Autodesk Inventor part; units mm, degrees
ref_plane "YZ Plane" through (0, 0, 0) normal (1, 0, 0) x (0, 1, 0)
ref_plane "XZ Plane" through (0, 0, 0) normal (0, 1, 0) x (-1, 0, 0)
ref_plane "XY Plane" through (0, 0, 0) normal (0, 0, 1) x (1, 0, 0)
sketch "草圖1" plane through (0, 0, 0) normal (0, 0, 1) x (1, 0, 0)
  circle A0 centre (0, 0) radius 32
  dimension "d0" = 64
extrude "擠出1" add sketch "草圖1" along normal blind 4.5
sketch "草圖2" plane through (0, 0, 4.5) normal (0, 0, 1) x (1, 0, 0)
  point P0 (0, 0)
  point P1 (0, 0)
hole "孔1" at (0, 0, 4.5) direction (0, 0, -1) diameter 30 end through all
sketch "草圖3" plane through (0, 0, 4.5) normal (0, 0, 1) x (1, 0, 0)
  circle A0 centre (15, 0) radius 2.15
  point P0 (0, 0)
  dimension "d10" = 0
  dimension "d11" = 4.3
  dimension "d12" = 15
extrude "擠出2" cut sketch "草圖3" against normal blind 20
pattern_circular "環形陣列1" count 2 over 360 about axis through (0, 0, -86.1215) along (0, 0, 1) of "擠出2"
properties part number "銅墊塊-50T"
Read the model definition and answer for the solid it produces. Units are mm, in the model's axes. A direction names the side the tool comes from. Round coordinates to 2 decimals unless told otherwise and drop trailing zeros. Write each loop counter-clockwise with the first axis right and the second up, starting at its lowest first coordinate (ties: lowest second). Pieces come first, ordered by that corner, then holes. Notation, with made-up numbers: (43, -14.5) - (66, -14.5) arc R29 ccw to (66, 5.5) - close; hole circle Ø1 at (-32.75, -29.75). An arc over 180 degrees is marked (long way). One line per question, with ' | ' between items. Start each with the question number.
1. For a pull along X with two mould halves and no side action, classify faces 3 (the face through (-17.15, 0.05, 2.28)), 4 (the face through (14, -7, 0)), 5 (the face through (-6.94, 31.24, 2.22)), 6 (the face through (0, -15, 2)) as +X half, -X half, draft (parallel to the pull), parting line (faces both ways), or undercut.
2. Section C-C (z = 1.85) is taken. Determine the outline of the cut face in (x, y), and give its area (3 significant figures).
3. This flat-tipped pin is pushed along its axis until it touches: pin 1 (1.5 mm diameter, centred on x = 11.5, z = 3.5, fed in from +Y). Where does it stop, or does it pass through?
4. For faces 1 (the face through (0, 15, 2)), 2 (the face through (14, -7, 4.5)), determine the directions among +Z, -Z, +X, -X, +Y, -Y from which every point of the face is accessible in a straight line to the end or side of a thin tool.
5. Section A-A (y = 0) is taken. Determine the outline of the cut face in (x, z), and give its area (3 significant figures).
6. Section B-B (x = 0) is taken. Determine the outline of the cut face in (y, z).
7. Section D-D (x = 20) is taken. Determine the outline of the cut face in (y, z).
8. Find the intervals of material crossed by probe 1 along X at (y, z) = (11.5, 1.15); probe 2 along Y at (x, z) = (-5, 2.05); probe 3 along Y at (x, z) = (-16, 2.8), in increasing order. Write a range as [from, to].
Filled in:
1) face 3: undercut | face 4: draft | face 5: parting line | face 6: undercut
2) outline: circle Ø64 at (0, 0); hole (-14.85, -2.14) arc R15 ccw to (14.85, -2.14) arc R2.15 ccw (long way) to (14.85, 2.14) arc R15 ccw to (-14.85, 2.14) arc R2.15 ccw (long way) to start | area: 2,500 mm²
3) pin 1: y = 30.14
4) face 1: +Z, -Z | face 2: +Z, +X, -X, +Y, -Y
5) outline: (-32, 0) - (-17.15, 0) - (-17.15, 4.5) - (-32, 4.5) - close; (17.15, 0) - (32, 0) - (32, 4.5) - (17.15, 4.5) - close | area: 134 mm²
6) outline: (-32, 0) - (-15, 0) - (-15, 4.5) - (-32, 4.5) - close; (15, 0) - (32, 0) - (32, 4.5) - (15, 4.5) - close
7) outline: (-24.98, 0) - (24.98, 0) - (24.98, 4.5) - (-24.98, 4.5) - close
8) probe 1: [-29.86, -9.63], [9.63, 29.86] | probe 2: [-31.61, -14.14], [14.14, 31.61] | probe 3: [-27.71, -1.9], [1.9, 27.71]
